```python
from build123d import *

# Parameters (mm, degrees)
SKETCH_W    = 80
SKETCH_H    = 95
SKETCH_R    = 3
PAD_DEPTH   = 10
FILLET_R    = 1
FILLET001_R = 1


with BuildPart() as part:
    # Sketch → Pad (new body)
    with BuildSketch(Plane.XY):
        with Locations((15, -18.5)):
            Rectangle(SKETCH_W, SKETCH_H)
        with Locations((-10, -52)):
            Circle(SKETCH_R, mode=Mode.SUBTRACT)
        with Locations((40, -52)):
            Circle(SKETCH_R, mode=Mode.SUBTRACT)
        with Locations((40, 22)):
            Circle(SKETCH_R, mode=Mode.SUBTRACT)
        with Locations((-10, 22)):
            Circle(SKETCH_R, mode=Mode.SUBTRACT)
        with BuildLine():
            ThreePointArc((-5, -6.244998), (8, 0), (-5, 6.244998))
            Line((-5, 6.244998), (-5, 10))
            ThreePointArc((-5, 10), (-7, 12), (-9, 10))
            Line((-9, 10), (-9, -10))
            ThreePointArc((-9, -10), (-7, -12), (-5, -10))
            Line((-5, -6.244998), (-5, -10))
        make_face(mode=Mode.SUBTRACT)
    extrude(amount=PAD_DEPTH)

    # Fillet
    fillet_edges = [part.edges().sort_by_distance(p)[0] for p in [
        (-25, -66, 5),
        (-25, 29, 5),
    ]]
    fillet(fillet_edges, radius=FILLET_R)

    # Fillet001
    fillet001_edges = [part.edges().sort_by_distance(p)[0] for p in [
        (55, -66, 5),
        (55, 29, 5),
    ]]
    fillet(fillet001_edges, radius=FILLET001_R)


solid = part.part
```
CAD build for the part. Positions are in the model's coordinates, mm. A direction names the side the tool comes from. Coordinates: 2 decimals unless noted, no trailing zeros. Write each loop counter-clockwise with the first axis right and the second up, starting at its lowest first coordinate (ties: lowest second). Pieces come first, ordered by that corner, then holes. Notation, with made-up numbers: (42, 17.25) -> (86, 17.25) arc R34 cw to (86, 56.25) -> close; hole circle Ø4 at (84.5, -26). An arc over 180 degrees is marked (long way). Return JSON: item names as keys, results as strings. Group by question number.
Q1. Cut at C-C, the plane z = 4. Give the cut face in (x, y) (3 decimals).
Q2. Which spindle directions (+Z, -Z, +X, -X, +Y, -Y) get a long thin tool onto all of the face, cutting with end or side? Do faces 4 (the face through (14, -18, 10)), 5 (the face through (-5, 8, 5)). Say none if no direction does.
Q3. Cut at A-A, the plane y = 0. Give the cut face in (x, z).
Q4. Cut at B-B, the plane x = -10. Give the cut face in (y, z), then the cut area to 3 significant figures.
Q5. Cut at D-D, the plane y = -52. Give the cut face in (x, z).
Q6. Drill centre lines: line 1 (Y direction, x = 40, z = 4.75); line 2 (X direction, y = 0, z = 5.75); line 3 (Y direction, x = 38, z = 0.5). Where is each one in solid material? Low to high.
Q7. Pull direction X, two halves, no side cores. Call faces 1 (the face through (55, -19, 5)), 2 (the face through (14, 29, 5)), 3 (the face through (37.79, -49.97, 4.93)): released by +X, released by -X, zero draft, split by the parting line, or undercut.
Returned:
{
 "1": {"outline": "(-25, -65) arc R1 ccw to (-24, -66) -> (54, -66) arc R1 ccw to (55, -65) -> (55, 28) arc R1 ccw to (54, 29) -> (-24, 29) arc R1 ccw to (-25, 28) -> close; hole circle Ø6 at (-10, -52); hole circle Ø6 at (-10, 22); hole (-9, -10) arc R2 ccw to (-5, -10) -> (-5, -6.245) arc R8 ccw (long way) to (-5, 6.245) -> (-5, 10) arc R2 ccw to (-9, 10) -> close; hole circle Ø6 at (40, -52); hole circle Ø6 at (40, 22)"},
 "2": {"face 4": "+Z, +X, -X, +Y, -Y", "face 5": "+Z, -Z"},
 "3": {"outline": "(-25, 0) -> (-9, 0) -> (-9, 10) -> (-25, 10) -> close; (8, 0) -> (55, 0) -> (55, 10) -> (8, 10) -> close"},
 "4": {"outline": "(-66, 0) -> (-55, 0) -> (-55, 10) -> (-66, 10) -> close; (-49, 0) -> (19, 0) -> (19, 10) -> (-49, 10) -> close; (25, 0) -> (29, 0) -> (29, 10) -> (25, 10) -> close", "area": "830 mm2"},
 "5": {"outline": "(-25, 0) -> (-13, 0) -> (-13, 10) -> (-25, 10) -> close; (-7, 0) -> (37, 0) -> (37, 10) -> (-7, 10) -> close; (43, 0) -> (55, 0) -> (55, 10) -> (43, 10) -> close"},
 "6": {"line 1": "y = -66 to -55, -49 to 19, 25 to 29", "line 2": "x = -25 to -9, 8 to 55", "line 3": "y = -66 to -54.24, -49.76 to 19.76, 24.24 to 29"},
 "7": {"face 1": "released by +X", "face 2": "zero draft", "face 3": "undercut"}
}
